Design review of the part built by this model. Coordinates are the model's own, in mm. Face numbers are marked on the shaded views. Give positions to 0.01 mm unless a question says otherwise; leave off trailing zeros. Order: outer loops, then holes, each group sorted by start corner. A loop starts at its lowest first (then second) coordinate and runs counter-clockwise, first axis right, second up.
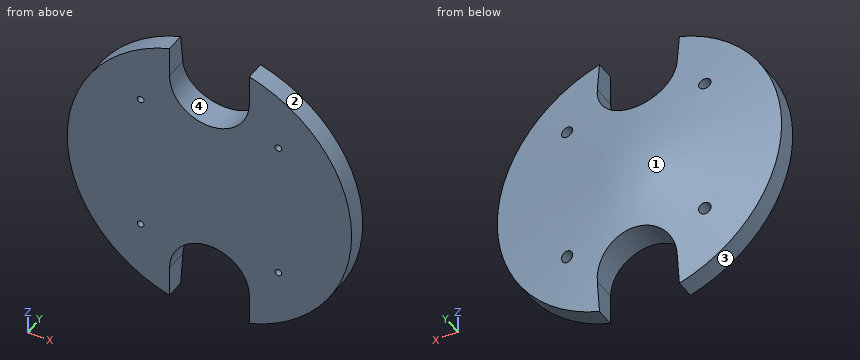
```python
from build123d import *

# Parameters (mm, degrees)
SKETCH4_R          = 1.7
CUT_EXTRUDE1_DEPTH = 106.157025443
CUT_EXTRUDE2_DEPTH = 106.157025601
SKETCH9_R          = 3
CUT_EXTRUDE3_DEPTH = 103.287584934


with BuildPart() as part:
    # Sketch2 → Revolve1 (revolve)
    with BuildSketch(Plane(origin=(0, 0, 0), x_dir=(0, 0, -1), z_dir=(1, 0, 0))):
        Polygon((0, 0), (73, 0), (73, 10), (0, 20), align=None)
    revolve(axis=Axis((0, 10, 0), (0, 1, 0)))

    # Sketch4 → Cut-Extrude1 (cut, through all)
    with BuildSketch(Plane.XZ):
        with Locations(Location((-35.355339059, 35.355339059, 0), (0, 0, 270))):
            Circle(SKETCH4_R)
        with Locations(Location((35.355339059, 35.355339059, 0), (0, 0, 270))):
            Circle(SKETCH4_R)
        with Locations(Location((35.355339059, -35.355339059, 0), (0, 0, 270))):
            Circle(SKETCH4_R)
        with Locations(Location((-35.355339059, -35.355339059, 0), (0, 0, 270))):
            Circle(SKETCH4_R)
    extrude(amount=-CUT_EXTRUDE1_DEPTH, mode=Mode.SUBTRACT)

    # Sketch5 → Cut-Extrude2 (cut, through all)
    with BuildSketch(Plane.XZ):
        with BuildLine():
            Line((-20.5, 54.5), (-20.5, 75))
            Line((-20.5, 75), (0, 75))
            Line((0, 75), (20.5, 75))
            Line((20.5, 75), (20.5, 54.5))
            ThreePointArc((20.5, 54.5), (0, 34), (-20.5, 54.5))
        make_face()
    cut_extrude2 = extrude(amount=-CUT_EXTRUDE2_DEPTH, mode=Mode.SUBTRACT)

    # Mirror1: Cut-Extrude2 across plane
    add(cut_extrude2.mirror(Plane.XY), mode=Mode.SUBTRACT)

    # Sketch9 → Cut-Extrude3 (cut, through all)
    with BuildSketch(Plane(origin=(0, 5, 0), x_dir=(1, 0, 0), z_dir=(0, 1, 0))):
        with Locations(Location((-35.355339059, -35.355339059, 0), (0, 0, 133.431744149))):
            Circle(SKETCH9_R)
        with Locations(Location((-35.355339059, 35.355339059, 0), (0, 0, 135))):
            Circle(SKETCH9_R)
        with Locations(Location((35.355339059, 35.355339059, 0), (0, 0, 136.568255851))):
            Circle(SKETCH9_R)
        with Locations(Location((35.355339059, -35.355339059, 0), (0, 0, 135))):
            Circle(SKETCH9_R)
    extrude(amount=CUT_EXTRUDE3_DEPTH, mode=Mode.SUBTRACT)


solid = part.part
```
1. Draft analysis for pull direction X (two halves, no side actions). For the marked faces 1, 2, 3 and 4, state which applies: pulls with the +X half, pulls with the -X half, needs draft (parallel to the pull), parting line crosses it, or undercut.
Recorded:
face 1: parting line crosses it
face 2: pulls with the +X half
face 3: pulls with the -X half
face 4: undercut
2. For line 1 along Y through (x, z) = (-52, -26); line 2 along X through (y, z) = (5, 53); line 3 along X through (y, z) = (9.75, -60.5), list the stretches that pass through material, from the lowest coordinate up.
Recorded:
line 1: y = 0 to 12.04
line 2: x = -50.2 to -20.45, 20.45 to 50.2
line 3: x = -40.85 to -20.5, 20.5 to 40.85
3. Take a section at A-A (y = 17). State the section outline as (x, z) points.
Recorded:
outline: circle Ø43.8 at (0, 0)
4. For pin 1 (7 mm diameter, centred on x = 35.36, z = 35.36, fed in from +Y); pin 2 (2.5 mm diameter, centred on x = -35.36, z = 35.36, fed in from +Y); pin 3 (1.5 mm diameter, centred on y = 8.5, z = 2, fed in from -X); pin 4 (4 mm diameter, centred on y = 9, z = -15.5, fed in from -X), all flat-tipped, find the tip position at first contact; note any pin that passes through.
Recorded:
pin 1: stops at y = 13.63
pin 2: passes through
pin 3: stops at x = -72.99
pin 4: stops at x = -71.74
